from build123d import *

# Parameters (mm, degrees)
SKETCH1_W                 = 44.1625
SKETCH1_H                 = 19.05
BOSS_EXTRUDE1_DEPTH       = 6.35
SKETCH2_W                 = 19.05
SKETCH2_H                 = 19.05
BOSS_EXTRUDE2_DEPTH       = 9.525
M8X1_0_TAPPED_HOLE1_D     = 7
M8X1_0_TAPPED_HOLE1_DEPTH = 21.082
M8X1_0_TAPPED_HOLE1_TIP   = 2.103012167
M8_CLEARANCE_HOLE1_D      = 9
M8_CLEARANCE_HOLE1_DEPTH  = 21.082
M8_CLEARANCE_HOLE1_TIP    = 2.703872786


with BuildPart() as part:
    # Sketch1 → Boss-Extrude1 (new body)
    with BuildSketch(Plane.XY):
        with Locations((38.24375, 204.55)):
            Rectangle(SKETCH1_W, SKETCH1_H)
    extrude(amount=BOSS_EXTRUDE1_DEPTH)

    # Sketch2 → Boss-Extrude2 (add, symmetric)
    with BuildSketch(Plane.XY.offset(6.35)):
        with Locations((25.6875, 204.55)):
            Rectangle(SKETCH2_W, SKETCH2_H)
    extrude(amount=BOSS_EXTRUDE2_DEPTH, both=True)

    # M8x1.0 Tapped Hole1
    with Locations(Plane(origin=(0, 214.075, 0), x_dir=(1, 0, 0), z_dir=(0, 1, 0))):
        with Locations((25.6875, -6.35)):
            Hole(M8X1_0_TAPPED_HOLE1_D / 2, depth=M8X1_0_TAPPED_HOLE1_DEPTH)
            with Locations((0, 0, -(M8X1_0_TAPPED_HOLE1_DEPTH + M8X1_0_TAPPED_HOLE1_TIP / 2))):  # 118° drill point
                Cone(0, M8X1_0_TAPPED_HOLE1_D / 2, M8X1_0_TAPPED_HOLE1_TIP, mode=Mode.SUBTRACT)

    # M8 Clearance Hole1
    with Locations(Plane.XY.offset(6.35)):
        with Locations((50.8, 204.55)):
            Hole(M8_CLEARANCE_HOLE1_D / 2, depth=M8_CLEARANCE_HOLE1_DEPTH)
            with Locations((0, 0, -(M8_CLEARANCE_HOLE1_DEPTH + M8_CLEARANCE_HOLE1_TIP / 2))):  # 118° drill point
                Cone(0, M8_CLEARANCE_HOLE1_D / 2, M8_CLEARANCE_HOLE1_TIP, mode=Mode.SUBTRACT)


solid = part.part
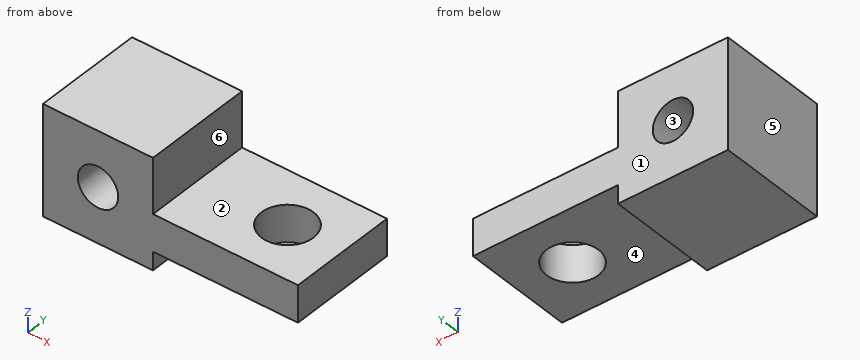
Verification items for the finished model (mm, model axes). Face numbers are marked on the shaded views. A direction names the side the tool comes from. Give positions to 0.01 mm unless a question says otherwise; leave off trailing zeros. Write each loop counter-clockwise with the first axis right and the second up, starting at its lowest first coordinate (ties: lowest second). Pieces come first, ordered by that corner, then holes. Notation, with made-up numbers: M 32.5,37.5 L 51.5,37.5 A20 ccw 51.5,66.5 Z; hole C 52,14.25 d5. An arc over 180 degrees is marked long. Use CSV: the item, a comma, the result in double quotes.
1) Access from +Z, -Z, +X, -X, +Y, -Y to the whole of each face (thin tool, end or side, straight path). Record for the marked faces 5 and 6.
Final values:
face 5,"+Z, -Z, -X, +Y, -Y"
face 6,"+Z, +X, +Y, -Y"
2) Release check for a two-part mould opening along Z. For the marked faces 1, 2, 3 and 4 record: released by +Z, released by -Z, zero draft, split by the parting line, or undercut.
Final values:
face 1,"zero draft"
face 2,"released by +Z"
face 3,"undercut"
face 4,"released by -Z"
3) Go/stop test with flat-tipped pins: pin 1 Ø3 at (x, y) = (44, 204.5) entering from +Z; pin 2 Ø10.5 at (y, z) = (202.5, 12) entering from +X; pin 3 Ø9.5 at (x, y) = (48, 208.5) entering from -Z. Record where each tip stops, or that it passes through.
Final values:
pin 1,"z = 6.35"
pin 2,"x = 35.21"
pin 3,"z = 0"
4) Cross-section at A-A (y = 204.55). State how many separate pieces and enclosed holes the cut face has, plus the area to 3 significant figures.
Final values:
separate pieces,"2"
enclosed holes,"1"
area,"427 mm²"
5) Cross-section at B-B (x = 50.8). Enter the section's corners in (y, z) (3 decimals), plus the area to 3 significant figures.
Final values:
outline,"M 195.025,0 L 200.05,0 L 200.05,6.35 L 195.025,6.35 Z; M 209.05,0 L 214.075,0 L 214.075,6.35 L 209.05,6.35 Z"
area,"63.8 mm²"
6) Material ranges on line 1 along X through (y, z) = (206, 4.5) (1 decimal); line 2 along Y through (x, z) = (50.8, 2.25) (3 decimals); line 3 along X through (y, z) = (208, 5.5) (1 decimal), recorded low to high.
Final values:
line 1,"16.2 to 22.7, 28.7 to 46.5, 55.1 to 60.3"
line 2,"195.025 to 200.05, 209.05 to 214.075"
line 3,"16.2 to 22.3, 29.1 to 47.9, 53.7 to 60.3"
